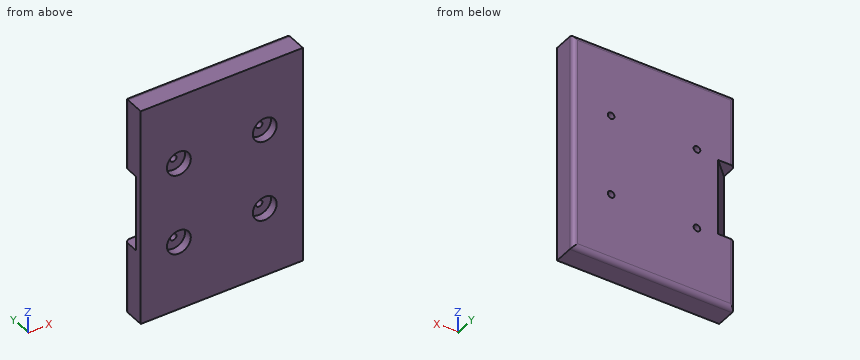
Autodesk Inventor part; units mm, degrees
ref_plane "YZ Plane" through (0, 0, 0) normal (1, 0, 0) x (0, 1, 0)
ref_plane "XZ Plane" through (0, 0, 0) normal (0, 1, 0) x (-1, 0, 0)
ref_plane "XY Plane" through (0, 0, 0) normal (0, 0, 1) x (1, 0, 0)
sketch "Sketch1" plane through (0, 0, 0) normal (0, 1, 0) x (-1, 0, 0)
  line L0 (85, 115) -> (-85, 115)
  line L1 (-85, 115) -> (-85, -115)
  line L2 (-85, -115) -> (85, -115)
  line L3 (85, -115) -> (85, 115)
  line L4 (85, 115) -> (-85, -115) construction
  line L5 (-85, 115) -> (85, -115) construction
  line L6 (-85, 115) -> (-85, 42.5) construction
  line L7 (-85, 42.5) -> (-85, -42.5) construction
  line L8 (-85, 42.5) -> (-45, 42.5) construction
  line L9 (-45, 42.5) -> (45, 42.5) construction
  line L10 (45, 42.5) -> (45, -42.5) construction
  line L11 (-85, -42.5) -> (-45, -42.5) construction
  line L12 (-45, -42.5) -> (45, -42.5) construction
  circle A0 centre (-45, 42.5) radius 3.5
  circle A1 centre (45, 42.5) radius 3.5
  circle A2 centre (45, -42.5) radius 3.5
  line L13 (-45, 42.5) -> (-45, -42.5) construction
  circle A3 centre (-45, -42.5) radius 3.5
  point P0 (0, 0)
  dimension "d3" = 85
  dimension "d7" = 7
  dimension "d8" = 7
extrude "Extrusion1" add sketch "Sketch1" along normal blind 25
sketch "Sketch2" plane through (0, 0, 0) normal (0, -1, 0) x (1, 0, 0)
  circle A0 centre (-45, -42.5) radius 3.5
  circle A1 centre (-45, -42.5) radius 12.5
  circle A2 centre (-45, 42.5) radius 3.5
  circle A3 centre (-45, 42.5) radius 12.5
  circle A4 centre (45, 42.5) radius 3.5
  circle A5 centre (45, 42.5) radius 12.5
  circle A6 centre (45, -42.5) radius 3.5
  circle A7 centre (45, -42.5) radius 12.5
  point P0 (0, 0)
extrude "Extrusion2" cut sketch "Sketch2" against normal blind 9
sketch "Sketch3" plane through (-85, 0, 115) normal (0, 0, 1) x (1, 0, 0)
  point P0 (85, 0)
sketch "Sketch4" plane through (0, 0, 0) normal (0, 0, 1) x (1, 0, 0)
  line L0 (-85, 0) -> (-85, 25)
  line L1 (-85, 7.3168) -> (-67.3168, 25)
  line L2 (-85, 25) -> (85, 25)
  line L3 (-85, 7.3168) -> (-59.9922, 7.3168) construction
  point P0 (0, 0)
  dimension "d15" = 45
extrude "Extrusion3" cut sketch "Sketch4" along normal mid plane 80
fillet "Fillet1" radius 5 5 edges at (85, 25, 0) (0, 25, 115) (-85, 25, 77.5) (-85, 25, -77.5) (0, 25, -115)
properties part number "Base"
The listing builds one solid part. Answer for the finished solid, in the listing's coordinates (mm). Coordinates: 2 decimals unless noted, no trailing zeros. Write each loop counter-clockwise with the first axis right and the second up, starting at its lowest first coordinate (ties: lowest second). Pieces come first, ordered by that corner, then holes. Notation, with made-up numbers: (7, -34) - (56, -34) arc R20 cw to (56, -17) - close; hole circle Ø10 at (64, 77). An arc over 180 degrees is marked (long way). Return JSON: item names as keys, results as strings.
1. Consider line 1 along Z through (x, y) = (-45, 17); line 2 along Z through (x, y) = (-45, 6.75); line 3 along X through (y, z) = (20.5, 74.5). Determine where each line is inside the solid, lowest interval first.
Final values:
{"line 1": "-115 to -46, -39 to 39, 46 to 115", "line 2": "-115 to -55, -30 to 30, 55 to 115", "line 3": "-84.97 to 84.97"}
2. The part is cut by section B-B on x = -45. Determine the outline of the cut face in (y, z).
Final values:
{"outline": "(0, -115) - (20, -115) arc R5 ccw to (25, -110) - (25, -46) - (9, -46) - (9, -55) - (0, -55) - close; (0, -30) - (9, -30) - (9, -39) - (25, -39) - (25, 39) - (9, 39) - (9, 30) - (0, 30) - close; (0, 55) - (9, 55) - (9, 46) - (25, 46) - (25, 110) arc R5 ccw to (20, 115) - (0, 115) - close"}
3. The part is cut by section A-A on z = 42.5. Determine the outline of the cut face in (x, y).
Final values:
{"outline": "(-85, 0) - (-57.5, 0) - (-57.5, 9) - (-48.5, 9) - (-48.5, 25) - (-80, 25) arc R5 ccw to (-85, 20) - close; (-41.5, 9) - (-32.5, 9) - (-32.5, 0) - (32.5, 0) - (32.5, 9) - (41.5, 9) - (41.5, 25) - (-41.5, 25) - close; (48.5, 9) - (57.5, 9) - (57.5, 0) - (85, 0) - (85, 20) arc R5 ccw to (80, 25) - (48.5, 25) - close"}
4. The part is cut by section C-C on z = -22. Determine the outline of the cut face in (x, y), then the cut area to 3 significant figures.
Final values:
{"outline": "(-85, 0) - (85, 0) - (85, 20) arc R5 ccw to (80, 25) - (-67.32, 25) - (-85, 7.32) - close", "area": "4,090 mm^2"}
5. Each of these flat-tipped pins is pushed along its axis until it touches: pin 1 Ø4 at (x, z) = (45, 42.5) entering from +Y; pin 2 Ø15 at (x, z) = (-45, 42.5) entering from -Y. Where does it stop, or does it pass through?
Final values:
{"pin 1": "through", "pin 2": "y = 9"}
